Part model, mm, in its own coordinate system. Coordinates: 2 decimals unless noted, no trailing zeros. Write each loop counter-clockwise with the first axis right and the second up, starting at its lowest first coordinate (ties: lowest second). Pieces come first, ordered by that corner, then holes. Notation, with made-up numbers: M -35,33 L -22,33 A6 cw -22,40 Z; hole C 42.25,-10.5 d5. An arc over 180 degrees is marked long. Use a Markdown table: item, result. Add a question column.
Q1. Slice it at C-C on y = 20.5. Write the cut outline in (x, z), then the cut area to 3 significant figures.
Q2. Slice it at B-B on x = 10.75. Write the cut outline in (y, z).
Q3. Slice it at A-A on y = 9.1. Write the cut outline in (x, z).
Q4. Wall check: L1, parallel to Z at x = 5, y = 13.5. Give the ranges that are in metal, low to high. Write a range as from..to.
Q5. Pin check, flat tips, straight feed: pin 1 Ø11.5 at (x, y) = (8.5, 45.5) entering from +Z; pin 2 Ø5 at (x, y) = (16.5, 26.5) entering from -Z. Stop position of each tip, or through.
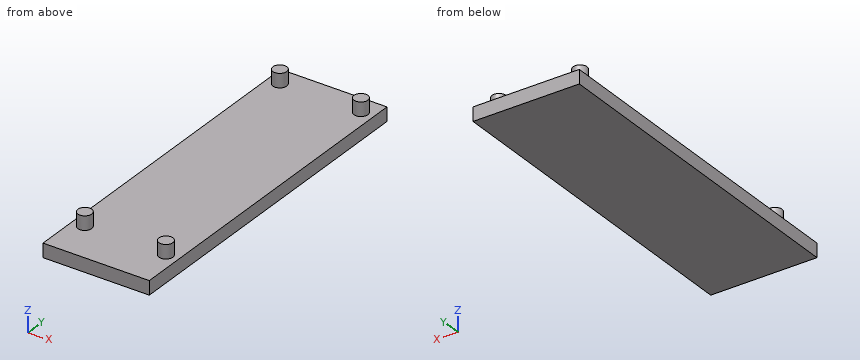
Autodesk Fusion 360 part; units mm, degrees
sketch "Sketch1" plane through (0, 0, 0) normal (0, 0, 1) x (1, 0, 0)
  line L0 (0, 0) -> (23, 0)
  line L1 (23, 0) -> (23, 74)
  line L2 (23, 74) -> (0, 74)
  line L3 (0, 74) -> (0, 0)
  dimension "d1" = 23
  dimension "d2" = 74
extrude "Extrude1" add sketch "Sketch1" along normal blind 3
sketch "Sketch2" plane through (0, 0, 3) normal (0, 0, 1) x (-1, 0, 0)
  line L0 (0, -74) -> (0, 0)
  line L1 (0, 0) -> (-23, 0)
  line L2 (-23, 0) -> (-23, -74)
  line L3 (-23, -74) -> (0, -74)
  circle A0 centre (-2.732, -9.1) radius 1.5
  circle A1 centre (-20.2682, -9.1) radius 1.5
  circle A2 centre (-2.732, -69.81) radius 1.5
  circle A3 centre (-20.2675, -69.81) radius 1.5
  dimension "d5" = 3
  dimension "d6" = 3
  dimension "d7" = 3
  dimension "d8" = 3
extrude "Extrude2" add sketch "Sketch2" along normal blind 3 contours A0 | A1 | A2 | A3
Recorded:
| question | item | result |
|---|---|---|
| 1 | outline | M 0,0 L 23,0 L 23,3 L 0,3 Z |
| 1 | area | 69.0 mm² |
| 2 | outline | M 0,0 L 74,0 L 74,3 L 0,3 Z |
| 3 | outline | M 0,0 L 23,0 L 23,3 L 21.77,3 L 21.77,6 L 18.77,6 L 18.77,3 L 4.23,3 L 4.23,6 L 1.23,6 L 1.23,3 L 0,3 Z |
| 4 | L1 | 0..3 |
| 5 | pin 1 | z = 3 |
| 5 | pin 2 | z = 0 |
